Input: part model. Units: mm. Frame: model coordinates. A direction names the side the tool comes from. Round coordinates to 2 decimals unless told otherwise and drop trailing zeros. Loops run counter-clockwise (first coordinate to the right, second up) from the corner with the lowest first, then second, coordinate; pieces in that order, holes last. Notation, with made-up numbers: M 22,8.5 L 36,8.5 A20 cw 36,32.5 Z; hole C -28.5,50 d5. An arc over 180 degrees is marked long. Return JSON: item names as keys, results as strings. Group by question number.
1) Section C-C (y = -8.75). Count the separate pieces of the cut face and the enclosed holes in it, plus the area to 3 significant figures.
2) Material intervals for line 1 (X direction, y = -9.75, z = 130); line 2 (Z direction, x = -133, y = -5); line 3 (Z direction, x = -164.5, y = -9.5), sorted ascending. Write a range as from..to.
3) Section B-B (z = 9.5). Output: boundary loops of the cut face in (x, y), plus the area to 3 significant figures.
4) Section A-A (x = -51). Output: boundary loops of the cut face in (y, z), plus the area to 3 significant figures.
5) Contact query for a flat-ended pin moving along its axis: P1, Ø5.5, axis at x = -33.5, z = -35, coming from the +Y side. Output: stop coordinate, or through.
6) Mould query, pull axis X, two halves, no side actions, for faces 4 (the face through (-84, -6, -43.023)), 5 (the face through (-267.15, -6.26, -186.99)), 6 (the face through (267.15, -6.26, 186.99)). Classes: +X half, -X half, draft (parallel to the pull), parting line (faces both ways), or undercut.
7) Access query for faces 1 (the face through (4, -12.7, -3)), 2 (the face through (-144.5, -6, 49)), 3 (the face through (-33, -3, -40)). Directions: +Z, -Z, +X, -X, +Y, -Y. A direction counts if a zero-diameter tool reaches every point of the face in a straight line with its end or side. Return the directions, or none.
from build123d import *

# Parameters (mm, degrees)
BOSS_EXTRUDE1_DEPTH         = 12.7
TAP_DRILL_FOR_1_4_20_TAP1_D = 5.1054
SKETCH10_R                  = 2.25
SKETCH10_R_2                = 2.2
CUT_EXTRUDE1_DEPTH          = 331.395656751
CUT_EXTRUDE2_REACH          = 332.396
SKETCH11_W                  = 88
SKETCH11_H                  = 11
SKETCH12_W                  = 40
SKETCH12_H                  = 272.22
CUT_EXTRUDE3_DEPTH          = 331.395656751
SKETCH13_W                  = 12
SKETCH13_H                  = 11
CUT_EXTRUDE4_DEPTH          = 3
FILLET2_R                   = 6.35
FILLET3_R                   = 3.175
SKETCH14_R                  = 2
CUT_EXTRUDE5_DEPTH          = 331.395656751


with BuildPart() as part:
    # Sketch1 → Boss-Extrude1 (new body)
    with BuildSketch(Plane(origin=(0, 0, 0), x_dir=(1, 0, 0), z_dir=(0, 1, 0))):
        with BuildLine():
            Line((-260, 190), (260, 190))
            ThreePointArc((260, 190), (267.071067812, 187.071067812), (270, 180))
            Line((270, 180), (270, -180))
            ThreePointArc((270, -180), (267.071067812, -187.071067812), (260, -190))
            Line((260, -190), (-260, -190))
            ThreePointArc((-260, -190), (-267.071067812, -187.071067812), (-270, -180))
            Line((-270, -180), (-270, 180))
            ThreePointArc((-270, 180), (-267.071067812, 187.071067812), (-260, 190))
        make_face()
    extrude(amount=-BOSS_EXTRUDE1_DEPTH)

    # Tap Drill for 1/4-20 Tap1 (through all)
    with Locations(Plane(origin=(0, 0, 0), x_dir=(1, 0, 0), z_dir=(0, 1, 0))):
        with Locations((-210, 130), (-210, -130), (210, 130), (210, -130)):
            Hole(TAP_DRILL_FOR_1_4_20_TAP1_D / 2)

    # Sketch10 → Cut-Extrude1 (cut, through all)
    with BuildSketch(Plane(origin=(0, 0, 0), x_dir=(1, 0, 0), z_dir=(0, 1, 0))):
        with Locations(Location((-137.95, -169.854932, 0), (0, 0, 270))):
            Circle(SKETCH10_R)
        with Locations(Location((-191.05, -169.854932, 0), (0, 0, 270))):
            Circle(SKETCH10_R)
        with Locations(Location((-133, 131.522913005, 0), (0, 0, 270))):
            Circle(SKETCH10_R_2)
        with Locations(Location((-33, 131.522913005, 0), (0, 0, 270))):
            Circle(SKETCH10_R_2)
        with Locations(Location((-133, 37.522913005, 0), (0, 0, 270))):
            Circle(SKETCH10_R_2)
        with Locations(Location((-33, 37.522913005, 0), (0, 0, 270))):
            Circle(SKETCH10_R_2)
    extrude(amount=-CUT_EXTRUDE1_DEPTH, mode=Mode.SUBTRACT)

    # Sketch11 → Cut-Extrude2 (cut, up to next)
    with BuildSketch(Plane(origin=(0, 0, 0), x_dir=(1, 0, 0), z_dir=(0, 1, 0)), mode=Mode.PRIVATE) as cut_extrude2_sk1:
        with Locations((-83, 37.522913005)):
            Rectangle(SKETCH11_W, SKETCH11_H)
    cut_extrude2_tool1 = extrude(cut_extrude2_sk1.sketch, amount=-CUT_EXTRUDE2_REACH, mode=Mode.PRIVATE) & part.part
    # Sketch11 → Cut-Extrude2 (cut, up to next)
    with BuildSketch(Plane(origin=(0, 0, 0), x_dir=(1, 0, 0), z_dir=(0, 1, 0)), mode=Mode.PRIVATE) as cut_extrude2_sk2:
        with Locations((-83, 131.522913005)):
            Rectangle(SKETCH11_W, SKETCH11_H)
    cut_extrude2_tool2 = extrude(cut_extrude2_sk2.sketch, amount=-CUT_EXTRUDE2_REACH, mode=Mode.PRIVATE) & part.part
    add(cut_extrude2_tool1.solids().sort_by_distance((-83, 0, -37.522913))[0], mode=Mode.SUBTRACT)
    add(cut_extrude2_tool2.solids().sort_by_distance((-83, 0, -131.522913))[0], mode=Mode.SUBTRACT)

    # Sketch12 → Cut-Extrude3 (cut, through all)
    with BuildSketch(Plane(origin=(0, 0, 0), x_dir=(1, 0, 0), z_dir=(0, 1, 0))):
        with Locations((-164.5, -47.569932)):
            Rectangle(SKETCH12_W, SKETCH12_H)
    extrude(amount=-CUT_EXTRUDE3_DEPTH, mode=Mode.SUBTRACT)

    # Sketch13 → Cut-Extrude4 (cut)
    with BuildSketch(Plane(origin=(0, 0, 0), x_dir=(1, 0, 0), z_dir=(0, 1, 0))):
        with Locations((-33, 37.522913005)):
            Rectangle(SKETCH13_W, SKETCH13_H)
        with Locations((-33, 131.522913005)):
            Rectangle(SKETCH13_W, SKETCH13_H)
        with Locations((-133, 37.522913005)):
            Rectangle(SKETCH13_W, SKETCH13_H)
        with Locations((-133, 131.522913005)):
            Rectangle(SKETCH13_W, SKETCH13_H)
    extrude(amount=-CUT_EXTRUDE4_DEPTH, mode=Mode.SUBTRACT)

    # Fillet2
    fillet2_edges = [part.edges().sort_by_distance(p)[0] for p in [
        (-144.5, -6.35, -88.540068),
        (-144.5, -6.35, 183.679932),
        (-184.5, -6.35, 183.679932),
        (-184.5, -6.35, -88.540068),
    ]]
    fillet(fillet2_edges, radius=FILLET2_R)

    # Fillet3
    fillet3_edges = [part.edges().sort_by_distance(p)[0] for p in [
        (-127, -7.85, -32.022913005),
        (-127, -7.85, -43.022913005),
        (-39, -7.85, -43.022913005),
        (-39, -7.85, -32.022913005),
        (-39, -7.85, -137.022913005),
        (-39, -7.85, -126.022913005),
        (-127, -7.85, -126.022913005),
        (-127, -7.85, -137.022913005),
        (-27, -1.5, -137.022913005),
        (-27, -1.5, -126.022913005),
        (-139, -1.5, -32.022913005),
        (-139, -1.5, -43.022913005),
        (-139, -1.5, -126.022913005),
        (-139, -1.5, -137.022913005),
        (-27, -1.5, -43.022913005),
        (-27, -1.5, -32.022913005),
    ]]
    fillet(fillet3_edges, radius=FILLET3_R)

    # Sketch14 → Cut-Extrude5 (cut, through all)
    with BuildSketch(Plane(origin=(0, 0, 0), x_dir=(1, 0, 0), z_dir=(0, 1, 0))):
        with Locations(Location((-164.5, 99.715068, 0), (0, 0, 270))):
            Circle(SKETCH14_R)
    extrude(amount=-CUT_EXTRUDE5_DEPTH, mode=Mode.SUBTRACT)


solid = part.part
Returned:
{
 "1": {"separate pieces": "1", "enclosed holes": "14", "area": "192,000 mm^2"},
 "2": {"line 1": "x = -270..-212.55, -207.45..-184.5, -144.5..207.45, 212.55..270", "line 2": "z = -190..-133.72, -129.32..-39.72, -35.32..190", "line 3": "z = -190..-101.72, -97.72..-88.54, 183.68..190"},
 "3": {"outline": "M -270,-12.7 L -184.5,-12.7 L -184.5,0 L -270,0 Z; M -144.5,-12.7 L 270,-12.7 L 270,0 L -144.5,0 Z", "area": "6,350 mm^2"},
 "4": {"outline": "M -12.7,-190 L 0,-190 L 0,-137.02 L -12.7,-137.02 Z; M -12.7,-126.02 L 0,-126.02 L 0,-43.02 L -12.7,-43.02 Z; M -12.7,-32.02 L 0,-32.02 L 0,190 L -12.7,190 Z", "area": "4,550 mm^2"},
 "5": {"P1": "stops at y = -3"},
 "6": {"face 4": "undercut", "face 5": "-X half", "face 6": "+X half"},
 "7": {"face 1": "+Z, -Z, +X, -X, -Y", "face 2": "+Y, -Y", "face 3": "+Y"}
}
